Input: part model. Units: mm. Frame: model coordinates. A direction names the side the tool comes from. Round coordinates to 2 decimals unless told otherwise and drop trailing zeros. Loops run counter-clockwise (first coordinate to the right, second up) from the corner with the lowest first, then second, coordinate; pieces in that order, holes last. Notation, with made-up numbers: (7, -38) -> (20, -38) arc R32 cw to (20, -8) -> close; hole circle Ø10 at (79, 44). An arc over 180 degrees is marked (long way). Answer as a JSON object with one key per item and string values. Group by question number.
Item 1: Draft query along X for faces 5 (the flat face through (22, 9, 31.5)), 6 (the cylindrical face through (7.18, 0.76, 19.08)), 7 (the flat face through (0, 1, 17)). Return one class per face: released by +X, released by -X, zero draft, split by the parting line, or undercut.
Item 2: Set-up query: faces 1 (the flat face through (30.5, 9, 9)), 2 (the flat face through (22, 9, 14.5)), 3 (the flat face through (22, 9, 2.5)), 4 (the flat face through (14, 9, 9)). Return all of +Z, -Z, +X, -X, +Y, -Y with unobstructed straight access to the full face (end or side cutting, diameter ignored); none if empty.
Item 3: Section query B-B on x = 35.88. Return loops of the section in (y, z), and give its area (4 significant figures).
Item 4: Material intervals for line 1 (X direction, y = 0.65, z = 17); line 2 (Z direction, x = 25, y = 7.5); line 3 (Y direction, x = 22, z = 32), sorted ascending. Write a range as [from, to].
Item 5: Pin query (flat end, axial travel): pin 1 (8 mm diameter, centred on x = 22.5, y = 8.5, fed in from +Z); pin 2 (4 mm diameter, centred on y = 13.5, z = 10.5, fed in from +X); pin 3 (6 mm diameter, centred on x = 8.04, z = 17, fed in from +Y). Return the tip coordinate at first contact, or that it passes through.
Item 6: Section query D-D on x = 19. Return loops of the section in (y, z), and give its area (3 significant figures).
Item 7: Section query C-C on z = 17. Return loops of the section in (x, y), and give its area (3 significant figures).
Item 8: Section query A-A on y = 12.5. Return loops of the section in (x, z), and give its area (3 significant figures).
from build123d import *

# Parameters (mm, degrees)
SKETCH1_W           = 50
SKETCH1_H           = 34
BOSS_EXTRUDE1_DEPTH = 1.5
FILLET1_R           = 12
SKETCH2_R           = 2.25
CUT_EXTRUDE1_DEPTH  = 1.5
SKETCH3_W           = 16.5
SKETCH3_H           = 12
BOSS_EXTRUDE2_DEPTH = 15.5


with BuildPart() as part:
    # Sketch1 → Boss-Extrude1 (new body)
    with BuildSketch(Plane(origin=(0, 0, 0), x_dir=(1, 0, 0), z_dir=(0, 1, 0))):
        with Locations((25, -17)):
            Rectangle(SKETCH1_W, SKETCH1_H)
    extrude(amount=BOSS_EXTRUDE1_DEPTH)

    # Fillet1
    fillet1_edges = [part.edges().sort_by_distance(p)[0] for p in [
        (0, 0.75, 0),
        (0, 0.75, 34),
    ]]
    fillet(fillet1_edges, radius=FILLET1_R)

    # Sketch2 → Cut-Extrude1 (cut)
    with BuildSketch(Plane(origin=(0, 1.5, 0), x_dir=(1, 0, 0), z_dir=(0, 1, 0))):
        with Locations(Location((8.04, -17, 0), (0, 0, 270))):
            Circle(SKETCH2_R)
        with Locations(Location((35.88, -17, 0), (0, 0, 270))):
            Circle(SKETCH2_R)
    extrude(amount=-CUT_EXTRUDE1_DEPTH, mode=Mode.SUBTRACT)

    # Sketch3 → Boss-Extrude2 (add)
    with BuildSketch(Plane(origin=(0, 1.5, 0), x_dir=(1, 0, 0), z_dir=(0, 1, 0))):
        with Locations((22.25, -8.5)):
            Rectangle(SKETCH3_W, SKETCH3_H)
        with Locations((22.25, -25.5)):
            Rectangle(SKETCH3_W, SKETCH3_H)
    extrude(amount=BOSS_EXTRUDE2_DEPTH)


solid = part.part
Solved:
{
 "1": {"face 5": "zero draft", "face 6": "undercut", "face 7": "released by -X"},
 "2": {"face 1": "+Z, -Z, +X, +Y", "face 2": "+X, -X, +Y", "face 3": "-Z, +X, -X, +Y", "face 4": "+Z, -Z, -X, +Y"},
 "3": {"outline": "(0, 0) -> (1.5, 0) -> (1.5, 14.75) -> (0, 14.75) -> close; (0, 19.25) -> (1.5, 19.25) -> (1.5, 34) -> (0, 34) -> close", "area": "44.25 mm²"},
 "4": {"line 1": "[0, 5.79], [10.29, 33.63], [38.13, 50]", "line 2": "[2.5, 14.5], [19.5, 31.5]", "line 3": "[0, 1.5]"},
 "5": {"pin 1": "z = 31.5", "pin 2": "x = 30.5", "pin 3": "y = 1.5"},
 "6": {"outline": "(0, 0) -> (1.5, 0) -> (1.5, 2.5) -> (17, 2.5) -> (17, 14.5) -> (1.5, 14.5) -> (1.5, 19.5) -> (17, 19.5) -> (17, 31.5) -> (1.5, 31.5) -> (1.5, 34) -> (0, 34) -> close", "area": "423 mm²"},
 "7": {"outline": "(0, 0) -> (5.79, 0) -> (5.79, 1.5) -> (0, 1.5) -> close; (10.29, 0) -> (33.63, 0) -> (33.63, 1.5) -> (10.29, 1.5) -> close; (38.13, 0) -> (50, 0) -> (50, 1.5) -> (38.13, 1.5) -> close", "area": "61.5 mm²"},
 "8": {"outline": "(14, 2.5) -> (30.5, 2.5) -> (30.5, 14.5) -> (14, 14.5) -> close; (14, 19.5) -> (30.5, 19.5) -> (30.5, 31.5) -> (14, 31.5) -> close", "area": "396 mm²"}
}
